from build123d import *

# Parameters (mm, degrees)
SKETCH1_R               = 24.07
BOSS_EXTRUDE1_DEPTH     = 2
BOSS_EXTRUDE2_DEPTH     = 5.5
BOSS_EXTRUDE5_REACH     = 36.482
SKETCH2_R               = 3
SKETCH1_5_R             = 34.31362745
CUT_EXTRUDE3_DEPTH      = 35.48158639
CUT_EXTRUDE3_DEPTH_BACK = 35.48158639
M2_5_CLEARANCE_HOLE1_D  = 2.7
CUT_EXTRUDE4_DEPTH      = 35.48158639


with BuildPart() as part:
    # Sketch1 → Boss-Extrude1 (new body)
    with BuildSketch(Plane(origin=(0, 0, 0), x_dir=(1, 0, 0), z_dir=(0, 1, 0))):
        with Locations(Location((0, 0, 0), (0, 0, 270))):
            Circle(SKETCH1_R)
    extrude(amount=BOSS_EXTRUDE1_DEPTH)

    # Sketch1<3> → Boss-Extrude2 (add)
    with BuildSketch(Plane(origin=(0, 0, 0), x_dir=(1, 0, 0), z_dir=(0, 1, 0))):
        with BuildLine():
            ThreePointArc((12.366915807, 20.650043424), (14.541516735, 19.180959075), (16.543257949, 17.483864459))
            Line((16.543257949, 17.483864459), (18.089781085, 19.118318867))
            Line((18.089781085, 19.118318867), (13.523019488, 22.580483607))
            Line((13.523019488, 22.580483607), (12.366915807, 20.650043424))
        make_face()
        with BuildLine():
            ThreePointArc((16.543257949, -17.483864459), (14.541516735, -19.180959075), (12.366915807, -20.650043424))
            Line((12.366915807, -20.650043424), (13.523019488, -22.580483607))
            Line((13.523019488, -22.580483607), (18.089781085, -19.118318867))
            Line((18.089781085, -19.118318867), (16.543257949, -17.483864459))
        make_face()
        with BuildLine():
            ThreePointArc((-16.543257949, 17.483864459), (-14.541516735, 19.180959075), (-12.366915807, 20.650043424))
            Line((-12.366915807, 20.650043424), (-13.523019488, 22.580483607))
            Line((-13.523019488, 22.580483607), (-18.089781085, 19.118318867))
            Line((-18.089781085, 19.118318867), (-16.543257949, 17.483864459))
        make_face()
        with BuildLine():
            ThreePointArc((-12.366915807, -20.650043424), (-14.541516735, -19.180959075), (-16.543257949, -17.483864459))
            Line((-16.543257949, -17.483864459), (-18.089781085, -19.118318867))
            Line((-18.089781085, -19.118318867), (-13.523019488, -22.580483607))
            Line((-13.523019488, -22.580483607), (-12.366915807, -20.650043424))
        make_face()
    extrude(amount=BOSS_EXTRUDE2_DEPTH)

    # Boss-Extrude5: up to this face of the body (flat: up to its plane)
    boss_extrude5_end = Plane(part.part.faces().sort_by_distance((15.168468653, 5.5, 20.00793877))[0])
    # Sketch2 → Boss-Extrude5 (add, up to the picked face)
    with BuildSketch(Plane(origin=(0, 0, 0), x_dir=(1, 0, 0), z_dir=(0, 1, 0)), mode=Mode.PRIVATE) as boss_extrude5_sk1:
        with Locations((13.97, 17.78)):
            Circle(SKETCH2_R)
    boss_extrude5_tool1 = split(extrude(boss_extrude5_sk1.sketch, amount=BOSS_EXTRUDE5_REACH, mode=Mode.PRIVATE), bisect_by=boss_extrude5_end, keep=Keep.BOTH, mode=Mode.PRIVATE)
    # Sketch2 → Boss-Extrude5 (add, up to the picked face)
    with BuildSketch(Plane(origin=(0, 0, 0), x_dir=(1, 0, 0), z_dir=(0, 1, 0)), mode=Mode.PRIVATE) as boss_extrude5_sk2:
        with Locations((13.97, -17.78)):
            Circle(SKETCH2_R)
    boss_extrude5_tool2 = split(extrude(boss_extrude5_sk2.sketch, amount=BOSS_EXTRUDE5_REACH, mode=Mode.PRIVATE), bisect_by=boss_extrude5_end, keep=Keep.BOTH, mode=Mode.PRIVATE)
    # Sketch2 → Boss-Extrude5 (add, up to the picked face)
    with BuildSketch(Plane(origin=(0, 0, 0), x_dir=(1, 0, 0), z_dir=(0, 1, 0)), mode=Mode.PRIVATE) as boss_extrude5_sk3:
        with Locations((-13.97, -17.78)):
            Circle(SKETCH2_R)
    boss_extrude5_tool3 = split(extrude(boss_extrude5_sk3.sketch, amount=BOSS_EXTRUDE5_REACH, mode=Mode.PRIVATE), bisect_by=boss_extrude5_end, keep=Keep.BOTH, mode=Mode.PRIVATE)
    # Sketch2 → Boss-Extrude5 (add, up to the picked face)
    with BuildSketch(Plane(origin=(0, 0, 0), x_dir=(1, 0, 0), z_dir=(0, 1, 0)), mode=Mode.PRIVATE) as boss_extrude5_sk4:
        with Locations((-13.97, 17.78)):
            Circle(SKETCH2_R)
    boss_extrude5_tool4 = split(extrude(boss_extrude5_sk4.sketch, amount=BOSS_EXTRUDE5_REACH, mode=Mode.PRIVATE), bisect_by=boss_extrude5_end, keep=Keep.BOTH, mode=Mode.PRIVATE)
    add(boss_extrude5_tool1.solids().sort_by(Axis((13.97, 0, -17.78), (0, 1, 0)))[0])
    add(boss_extrude5_tool2.solids().sort_by(Axis((13.97, 0, 17.78), (0, 1, 0)))[0])
    add(boss_extrude5_tool3.solids().sort_by(Axis((-13.97, 0, 17.78), (0, 1, 0)))[0])
    add(boss_extrude5_tool4.solids().sort_by(Axis((-13.97, 0, -17.78), (0, 1, 0)))[0])

    # Sketch1<5> → Cut-Extrude3 (cut, two sides)
    with BuildSketch(Plane(origin=(0, 0, 0), x_dir=(1, 0, 0), z_dir=(0, 1, 0))) as cut_extrude3_sk:
        Circle(SKETCH1_5_R)
        with BuildLine():
            Line((18.089781085, 19.118318867), (16.543257949, 17.483864459))
            ThreePointArc((16.543257949, 17.483864459), (22.108382108, 9.517580605), (24.07, 0))
            ThreePointArc((24.07, 0), (22.108382108, -9.517580605), (16.543257949, -17.483864459))
            Line((16.543257949, -17.483864459), (18.089781085, -19.118318867))
            Line((18.089781085, -19.118318867), (13.523019488, -22.580483607))
            Line((13.523019488, -22.580483607), (12.366915807, -20.650043424))
            ThreePointArc((12.366915807, -20.650043424), (0, -24.07), (-12.366915807, -20.650043424))
            Line((-12.366915807, -20.650043424), (-13.523019488, -22.580483607))
            Line((-13.523019488, -22.580483607), (-18.089781085, -19.118318867))
            Line((-18.089781085, -19.118318867), (-16.543257949, -17.483864459))
            ThreePointArc((-16.543257949, -17.483864459), (-24.07, 0), (-16.543257949, 17.483864459))
            Line((-16.543257949, 17.483864459), (-18.089781085, 19.118318867))
            Line((-18.089781085, 19.118318867), (-13.523019488, 22.580483607))
            Line((-13.523019488, 22.580483607), (-12.366915807, 20.650043424))
            ThreePointArc((-12.366915807, 20.650043424), (0, 24.07), (12.366915807, 20.650043424))
            Line((12.366915807, 20.650043424), (13.523019488, 22.580483607))
            Line((13.523019488, 22.580483607), (18.089781085, 19.118318867))
        make_face(mode=Mode.SUBTRACT)
    extrude(amount=CUT_EXTRUDE3_DEPTH, mode=Mode.SUBTRACT)
    extrude(cut_extrude3_sk.sketch, amount=-CUT_EXTRUDE3_DEPTH_BACK, mode=Mode.SUBTRACT)

    # M2.5 Clearance Hole1 (through all)
    with Locations(Plane(origin=(0, 5.5, 0), x_dir=(1, 0, 0), z_dir=(0, 1, 0))):
        with Locations((-13.97, 17.78), (13.97, 17.78), (13.97, -17.78), (-13.97, -17.78)):
            Hole(M2_5_CLEARANCE_HOLE1_D / 2)

    # Sketch8 → Cut-Extrude4 (cut, through all)
    with BuildSketch(Plane.XZ):
        with BuildLine():
            ThreePointArc((-12.157407277, 20.77407876), (-11.650071144, 20.400673597), (-11.217885814, 19.942375432))
            Line((-11.217885814, 19.942375432), (-10.477447975, 19))
            Line((-10.477447975, 19), (-4.5, 19))
            Line((-4.5, 19), (-4.5, 21))
            Line((-4.5, 21), (-7, 21))
            Line((-7, 21), (-7, 23))
            Line((-7, 23), (7, 23))
            Line((7, 23), (7, 21))
            Line((7, 21), (4.5, 21))
            Line((4.5, 21), (4.5, 19))
            Line((4.5, 19), (10.477447975, 19))
            Line((10.477447975, 19), (11.217885814, 19.942375432))
            ThreePointArc((11.217885814, 19.942375432), (11.650071144, 20.400673597), (12.157407277, 20.77407876))
            ThreePointArc((12.157407277, 20.77407876), (0, 24.07), (-12.157407277, 20.77407876))
        make_face()
        with BuildLine():
            Line((10, 7.062206513), (10, -7.062206513))
            Line((10, -7.062206513), (16.722114186, -15.617624568))
            ThreePointArc((16.722114186, -15.617624568), (17.065148682, -16.145969817), (17.307920228, -16.727247155))
            ThreePointArc((17.307920228, -16.727247155), (24.07, 0), (17.307920228, 16.727247155))
            ThreePointArc((17.307920228, 16.727247155), (17.065148682, 16.145969817), (16.722114186, 15.617624568))
            Line((16.722114186, 15.617624568), (10, 7.062206513))
        make_face()
        with BuildLine():
            Line((-10, -7.062206513), (-10, 7.062206513))
            Line((-10, 7.062206513), (-16.722114186, 15.617624568))
            ThreePointArc((-16.722114186, 15.617624568), (-17.065148682, 16.145969817), (-17.307920228, 16.727247155))
            ThreePointArc((-17.307920228, 16.727247155), (-24.07, 0), (-17.307920228, -16.727247155))
            ThreePointArc((-17.307920228, -16.727247155), (-17.065148682, -16.145969817), (-16.722114186, -15.617624568))
            Line((-16.722114186, -15.617624568), (-10, -7.062206513))
        make_face()
        with BuildLine():
            Line((11.217885814, -19.942375432), (10.477447975, -19))
            Line((10.477447975, -19), (4.5, -19))
            Line((4.5, -19), (4.5, -21))
            Line((4.5, -21), (7, -21))
            Line((7, -21), (7, -23))
            Line((7, -23), (-7, -23))
            Line((-7, -23), (-7, -21))
            Line((-7, -21), (-4.5, -21))
            Line((-4.5, -21), (-4.5, -19))
            Line((-4.5, -19), (-10.477447975, -19))
            Line((-10.477447975, -19), (-11.217885814, -19.942375432))
            ThreePointArc((-11.217885814, -19.942375432), (-11.650071144, -20.400673597), (-12.157407277, -20.77407876))
            ThreePointArc((-12.157407277, -20.77407876), (0, -24.07), (12.157407277, -20.77407876))
            ThreePointArc((12.157407277, -20.77407876), (11.650071144, -20.400673597), (11.217885814, -19.942375432))
        make_face()
    extrude(amount=-CUT_EXTRUDE4_DEPTH, mode=Mode.SUBTRACT)


solid = part.part
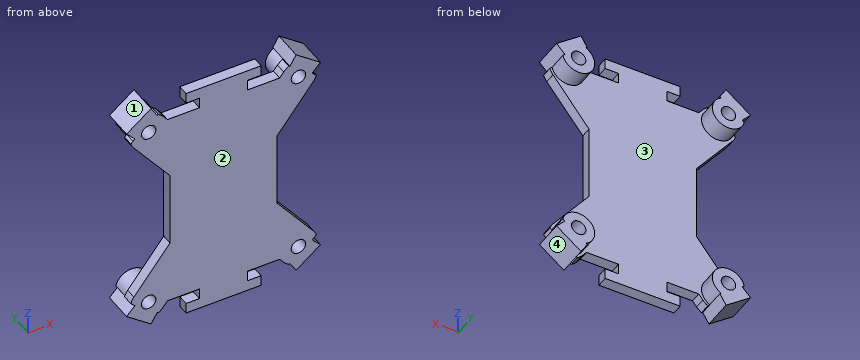
CAD build for the part. Positions are in the model's coordinates, mm. Face numbers are marked on the shaded views. Give positions to 0.01 mm unless a question says otherwise; leave off trailing zeros. Order: outer loops, then holes, each group sorted by start corner. A loop starts at its lowest first (then second) coordinate and runs counter-clockwise, first axis right, second up. Notation, with made-up numbers: (83.25, -11.5) -> (142.25, -11.5) arc R20 cw to (142.25, -7.5) -> close; hole circle Ø2 at (53, 85.25). An arc over 180 degrees is marked (long way). Return JSON: item names as keys, results as strings.
Q1. Saw through at A-A (y = 3.1). Write the cut outline in (x, z), then the cut area to 3 significant figures.
Working result:
{"outline": "(-18.09, -19.12) -> (-13.52, -22.58) -> (-12.37, -20.65) arc R24.07 cw to (-12.65, -20.48) arc R3 ccw (long way) to (-16.9, -17.14) arc R24.07 ccw to (-16.54, -17.48) -> close; (-18.09, 19.12) -> (-16.54, 17.48) arc R24.07 ccw to (-16.9, 17.14) arc R3 ccw (long way) to (-12.65, 20.48) arc R24.07 cw to (-12.37, 20.65) -> (-13.52, 22.58) -> close; (12.37, -20.65) -> (13.52, -22.58) -> (18.09, -19.12) -> (16.54, -17.48) arc R24.07 ccw to (16.9, -17.14) arc R3 ccw (long way) to (12.65, -20.48) arc R24.07 cw to start; (12.37, 20.65) arc R24.07 cw to (12.65, 20.48) arc R3 ccw (long way) to (16.9, 17.14) arc R24.07 ccw to (16.54, 17.48) -> (18.09, 19.12) -> (13.52, 22.58) -> close; hole circle Ø2.7 at (-13.97, -17.78); hole circle Ø2.7 at (-13.97, 17.78); hole circle Ø2.7 at (13.97, -17.78); hole circle Ø2.7 at (13.97, 17.78)", "area": "113 mm²"}
Q2. Saw through at D-D (z = 3.5). Write the cut outline in (x, y), then the cut area to 3 significant figures.
Working result:
{"outline": "(-10, 0) -> (10, 0) -> (10, 2) -> (-10, 2) -> close", "area": "40.0 mm²"}
Q3. Drill centre lines: line 1 (Z direction, x = 13.97, y = 4.15); line 2 (X direction, y = 1.3, z = -17.78); line 3 (Z direction, x = -13.97, y = 1.1). Where is each one in solid material? Low to high.
Working result:
{"line 1": "-22.24 to -19.13, -16.43 to -14.78, 14.78 to 16.43, 19.13 to 22.24", "line 2": "-16.82 to -15.32, -12.62 to 12.62, 15.32 to 16.82", "line 3": "-22.24 to -19.13, -16.43 to -12.11, 12.11 to 16.43, 19.13 to 22.24"}
Q4. Saw through at B-B (z = 18.5). Write the cut outline in (x, y), then the cut area to 3 significant figures.
Working result:
{"outline": "(-17.5, 0) -> (-15.11, 0) -> (-15.11, 5.5) -> (-17.5, 5.5) -> close; (-12.83, 0) -> (12.83, 0) -> (12.83, 5.5) -> (11.06, 5.5) -> (11.06, 2) -> (-11.06, 2) -> (-11.06, 5.5) -> (-12.83, 5.5) -> close; (15.11, 0) -> (17.5, 0) -> (17.5, 5.5) -> (15.11, 5.5) -> close", "area": "90.0 mm²"}
Q5. Mould opens along X. For the marked faces 1, 2, 3 and 4 say: pulls with the +X half, pulls with the -X half, needs draft (parallel to the pull), parting line crosses it, or undercut.
Working result:
{"face 1": "pulls with the -X half", "face 2": "needs draft", "face 3": "undercut", "face 4": "pulls with the +X half"}
Q6. Saw through at C-C (x = 7.5). Write the cut outline in (y, z).
Working result:
{"outline": "(0, -19) -> (2, -19) -> (2, 19) -> (0, 19) -> close"}
Q7. Flat gauge pins, fed straight in: pin 1 (1.5 mm diameter, centred on x = -6.5, z = -6.5, fed in from +Y); pin 2 (12 mm diameter, centred on x = 5.5, z = 18, fed in from -Y); pin 3 (0.6 mm diameter, centred on y = 0.5, z = 22.5, fed in from -X); pin 4 (1.6 mm diameter, centred on y = 1, z = 22, fed in from +X). Where does each tip first touch, or does it go through?
Working result:
{"pin 1": "y = 2", "pin 2": "y = 0", "pin 3": "x = -14.02", "pin 4": "x = 15.34"}
